Geometry: final body of the model. Coordinates: model frame, mm. A direction names the side the tool comes from. Round coordinates to 2 decimals unless told otherwise and drop trailing zeros. Loops run counter-clockwise (first coordinate to the right, second up) from the corner with the lowest first, then second, coordinate; pieces in that order, holes last. Notation, with made-up numbers: (72, 79) - (88, 79) arc R25 cw to (88, 114) - close; hole circle Ø3 at (45.25, 48.25). An arc over 180 degrees is marked (long way). Return JSON: item names as keys, results as strings. Group by question number.
1. Section A-A on x = -15. Return loops of the section in (y, z).
2. Material intervals for probe 1 along Y at (x, z) = (27, -3.1); probe 2 along X at (y, z) = (-23.5, -1.6); probe 3 along Y at (x, z) = (41.25, -1.55), sorted ascending.
3. Draft query along X for faces 1 (the face through (0, 12.5, 1)), 2 (the face through (-37.4, 5.86, -0.96)), 3 (the face through (-42, 5, -1)). Return one class per face: +X half, -X half, draft (parallel to the pull), parting line (faces both ways), or undercut.
4. Set-up query: faces 4 (the face through (-36.5, -17, -1)), 5 (the face through (0, 0, 0)), 6 (the face through (42, 5, -1)), 7 (the face through (-26, -25.5, 1)). Return all of +Z, -Z, +X, -X, +Y, -Y with unobstructed straight access to the full face (end or side cutting, diameter ignored); none if empty.
5. Section D-D on y = -12.5. Return loops of the section in (x, z).
6. Section B-B on y = 0. Return loops of the section in (x, z).
7. First-contact query: pin 1 Ø0.6 at (y, z) = (17.5, 1) entering from -X; pin 2 Ø3 at (y, z) = (3, -2) entering from +X; pin 3 Ø1.6 at (y, z) = (-7, 1.5) entering from +X; pin 4 Ø3 at (x, y) = (41.25, 0) entering from +Z. Flat tips, straight axial feed; report the tip coordinate or a pass-through.
8. Section C-C on z = -3. Return loops of the section in (x, y).
from build123d import *

# Parameters (mm, degrees)
F0_W     = 50
F0_H     = 7
F0_R     = 1.6
F1_DEPTH = 2
F2_DEPTH = 4
F3_SIZE  = 1.5
F4_R     = 3
F5_R     = 2


with BuildPart() as f1:
    # F0 (on Top) → F1 (new body)
    with BuildSketch(Plane.XY):
        with BuildLine():
            Line((-36.5, -5), (-36.5, 5))
            Line((-36.5, 5), (-44.577747, 5))
            ThreePointArc((-44.577747, 5), (-46, 0), (-44.577747, -5))
            Line((-44.577747, -5), (-36.5, -5))
        make_face()
        Polygon((-38.5, 1.587713), (-38.5, -1.587713), (-41.25, -3.175426), (-44, -1.587713), (-44, 1.587713), (-41.25, 3.175426), align=None, mode=Mode.SUBTRACT)
        Polygon((36.5, 28.5), (-36.5, 28.5), (-36.5, 5), (-36.5, -5), (-36.5, -28.5), (36.5, -28.5), (36.5, -5), (36.5, 5), align=None)
        Polygon((-34, 21.050253), (-34, 26), (-29.050253, 26), (29.050253, 26), (34, 26), (34, 21.050253), (34, -21.050253), (34, -26), (29.050253, -26), (-29.050253, -26), (-34, -26), (-34, -21.050253), align=None, mode=Mode.SUBTRACT)
        Polygon((29.050253, 26), (-29.050253, 26), (-34, 21.050253), (-34, -21.050253), (-30.5, -24.550253), (-30.5, 4.5), (-21.5, 4.5), (-21.5, -25.5), (-29.550253, -25.5), (-29.050253, -26), (29.050253, -26), (34, -21.050253), (34, 21.050253), align=None)
        with Locations((0, 16)):
            Rectangle(F0_W, F0_H, mode=Mode.SUBTRACT)
        with BuildLine():
            Line((44.577747, 5), (36.5, 5))
            Line((36.5, 5), (36.5, -5))
            Line((36.5, -5), (44.577747, -5))
            ThreePointArc((44.577747, -5), (46, 0), (44.577747, 5))
        make_face()
        Polygon((41.25, -3.175426), (38.5, -1.587713), (38.5, 1.587713), (41.25, 3.175426), (44, 1.587713), (44, -1.587713), align=None, mode=Mode.SUBTRACT)
        Polygon((-41.25, -3.175426), (-38.5, -1.587713), (-38.5, 1.587713), (-41.25, 3.175426), (-44, 1.587713), (-44, -1.587713), align=None)
        with Locations((-41.25, 0)):
            Circle(F0_R, mode=Mode.SUBTRACT)
        Polygon((38.5, 1.587713), (38.5, -1.587713), (41.25, -3.175426), (44, -1.587713), (44, 1.587713), (41.25, 3.175426), align=None)
        with Locations((41.25, 0)):
            Circle(F0_R, mode=Mode.SUBTRACT)
        Polygon((34, 26), (29.050253, 26), (34, 21.050253), align=None)
        Polygon((-29.050253, 26), (-34, 26), (-34, 21.050253), align=None)
        Polygon((-30.5, -24.550253), (-34, -21.050253), (-34, -26), (-29.050253, -26), (-29.550253, -25.5), (-30.5, -25.5), align=None)
        Polygon((34, -26), (34, -21.050253), (29.050253, -26), align=None)
    extrude(amount=F1_DEPTH)

    # F0 (on Top) → F2 (join)
    with BuildSketch(Plane.XY):
        Polygon((36.5, 28.5), (-36.5, 28.5), (-36.5, 5), (-36.5, -5), (-36.5, -28.5), (36.5, -28.5), (36.5, -5), (36.5, 5), align=None)
        Polygon((-34, 21.050253), (-34, 26), (-29.050253, 26), (29.050253, 26), (34, 26), (34, 21.050253), (34, -21.050253), (34, -26), (29.050253, -26), (-29.050253, -26), (-34, -26), (-34, -21.050253), align=None, mode=Mode.SUBTRACT)
        with BuildLine():
            Line((-36.5, -5), (-36.5, 5))
            Line((-36.5, 5), (-44.577747, 5))
            ThreePointArc((-44.577747, 5), (-46, 0), (-44.577747, -5))
            Line((-44.577747, -5), (-36.5, -5))
        make_face()
        Polygon((-38.5, 1.587713), (-38.5, -1.587713), (-41.25, -3.175426), (-44, -1.587713), (-44, 1.587713), (-41.25, 3.175426), align=None, mode=Mode.SUBTRACT)
        Polygon((-41.25, -3.175426), (-38.5, -1.587713), (-38.5, 1.587713), (-41.25, 3.175426), (-44, 1.587713), (-44, -1.587713), align=None)
        with Locations((-41.25, 0)):
            Circle(F0_R, mode=Mode.SUBTRACT)
        with BuildLine():
            Line((44.577747, 5), (36.5, 5))
            Line((36.5, 5), (36.5, -5))
            Line((36.5, -5), (44.577747, -5))
            ThreePointArc((44.577747, -5), (46, 0), (44.577747, 5))
        make_face()
        Polygon((41.25, -3.175426), (38.5, -1.587713), (38.5, 1.587713), (41.25, 3.175426), (44, 1.587713), (44, -1.587713), align=None, mode=Mode.SUBTRACT)
        Polygon((38.5, 1.587713), (38.5, -1.587713), (41.25, -3.175426), (44, -1.587713), (44, 1.587713), (41.25, 3.175426), align=None)
        with Locations((41.25, 0)):
            Circle(F0_R, mode=Mode.SUBTRACT)
    extrude(amount=-F2_DEPTH)

    # F3
    f3_edges = [f1.edges().sort_by_distance(p)[0] for p in [
        (-42.85, 0, 2),
        (39.65, 0, 2),
    ]]
    chamfer(f3_edges, length=F3_SIZE)

    # F4
    f4_edges = [f1.edges().sort_by_distance(p)[0] for p in [
        (-36.5, -5, -1),
        (-36.5, 5, -1),
        (36.5, -5, -1),
        (36.5, 5, -1),
    ]]
    fillet(f4_edges, radius=F4_R)

    # F5
    f5_edges = [f1.edges().sort_by_distance(p)[0] for p in [
        (36.5, 28.5, -1),
        (-36.5, 28.5, -1),
        (-36.5, -28.5, -1),
        (36.5, -28.5, -1),
    ]]
    fillet(f5_edges, radius=F5_R)


solid = f1.part
Taken from the geometry:
{
 "1": {"outline": "(-28.5, -4) - (-26, -4) - (-26, 0) - (12.5, 0) - (12.5, 2) - (-28.5, 2) - close; (19.5, 0) - (26, 0) - (26, -4) - (28.5, -4) - (28.5, 2) - (19.5, 2) - close"},
 "2": {"probe 1": "-28.5 to -26, 26 to 28.5", "probe 2": "-36.5 to -34, 34 to 36.5", "probe 3": "-5 to -1.6, 1.6 to 5"},
 "3": {"face 1": "undercut", "face 2": "-X half", "face 3": "draft"},
 "4": {"face 4": "+Z, -Z, -X, -Y", "face 5": "-Z", "face 6": "+Z, -Z, +X, +Y", "face 7": "+Z, -Z"},
 "5": {"outline": "(-36.5, -4) - (-34, -4) - (-34, 0) - (-30.5, 0) - (-30.5, 2) - (-36.5, 2) - close; (-21.5, 0) - (34, 0) - (34, -4) - (36.5, -4) - (36.5, 2) - (-21.5, 2) - close"},
 "6": {"outline": "(-46, -4) - (-42.85, -4) - (-42.85, 0.5) - (-44.35, 2) - (-46, 2) - close; (-39.65, -4) - (-34, -4) - (-34, 0) - (-30.5, 0) - (-30.5, 2) - (-38.15, 2) - (-39.65, 0.5) - close; (-21.5, 0) - (34, 0) - (34, -4) - (39.65, -4) - (39.65, 0.5) - (38.15, 2) - (-21.5, 2) - close; (42.85, -4) - (46, -4) - (46, 2) - (44.35, 2) - (42.85, 0.5) - close"},
 "7": {"pin 1": "x = -36.5", "pin 2": "x = 45.88", "pin 3": "x = 37.1", "pin 4": "through"},
 "8": {"outline": "(-44.58, -5) - (-39.5, -5) arc R3 cw to (-36.5, -8) - (-36.5, -26.5) arc R2 ccw to (-34.5, -28.5) - (34.5, -28.5) arc R2 ccw to (36.5, -26.5) - (36.5, -8) arc R3 cw to (39.5, -5) - (44.58, -5) arc R9.5 ccw to (44.58, 5) - (39.5, 5) arc R3 cw to (36.5, 8) - (36.5, 26.5) arc R2 ccw to (34.5, 28.5) - (-34.5, 28.5) arc R2 ccw to (-36.5, 26.5) - (-36.5, 8) arc R3 cw to (-39.5, 5) - (-44.58, 5) arc R9.5 ccw to start; hole circle Ø3.2 at (-41.25, 0); hole (-34, -26) - (34, -26) - (34, 26) - (-34, 26) - close; hole circle Ø3.2 at (41.25, 0)"}
}
